Here's how the part is built. I have some questions about the finished solid (model axes, mm). A direction names the side the tool comes from. Give positions to 0.01 mm unless a question says otherwise; leave off trailing zeros. Write each loop counter-clockwise with the first axis right and the second up, starting at its lowest first coordinate (ties: lowest second). Pieces come first, ordered by that corner, then holes. Notation, with made-up numbers: (-4.5, -37.5) -> (49.5, -37.5) arc R9 ccw to (49.5, -26.5) -> close; hole circle Ø7 at (5, -8.75). An arc over 180 degrees is marked (long way). Return JSON: item names as keys, results as strings.
from build123d import *

# Parameters (mm, degrees)
F1_DEPTH  = 43.0059846
F4_DEPTH  = 44.9897246
F5_R      = 1.98374
F6_R      = 3.69316
F7_SIZE   = 33.4809846
F8_R      = 11.2530001
F8_R_2    = 1.5
F9_DEPTH  = 1.70942
F10_R     = 1.8288
F11_DEPTH = 1.70942
F12_R     = 0.762


with BuildPart() as f1:
    # F0 (on Top) → F1 (new body)
    with BuildSketch(Plane.XY):
        Polygon((-1.70942, 0), (0, 0), (0, 46.9734646), (46.9734646, 46.9734646), (46.9734646, 0), (48.6828846, 0), (48.6828846, 48.6828846), (-1.70942, 48.6828846), align=None)
    extrude(amount=F1_DEPTH)

    # F3 (on face) → F4 (join, through all)
    with BuildSketch(Plane.XZ):
        Polygon((48.6828846, 0), (46.9734646, 0), (46.9734646, -3.69316), (58.6041246, -3.69316), (58.6041246, -1.98374), (48.6828846, -1.98374), align=None)
        Polygon((0, 0), (-1.70942, 0), (-1.70942, -1.98374), (-11.63066, -1.98374), (-11.63066, -3.69316), (0, -3.69316), align=None)
    extrude(amount=-F4_DEPTH)

    # F5
    f5_edges = [f1.edges().sort_by_distance(p)[0] for p in [
        (0, 46.973465, 21.502992),
        (46.973465, 46.973465, 21.502992),
        (-1.70942, 22.494862, -1.98374),
        (48.682885, 22.494862, -1.98374),
    ]]
    fillet(f5_edges, radius=F5_R)

    # F6
    f6_edges = [f1.edges().sort_by_distance(p)[0] for p in [
        (48.682885, 48.682885, 21.502992),
        (-1.70942, 48.682885, 21.502992),
        (0, 22.494862, -3.69316),
        (46.973465, 22.494862, -3.69316),
    ]]
    fillet(f6_edges, radius=F6_R)

    # F7
    f7_edges = [f1.edges().sort_by_distance(p)[0] for p in [
        (-0.85471, 0, 43.005985),
        (47.828175, 0, 43.005985),
    ]]
    chamfer(f7_edges, length=F7_SIZE)

    # F8 (on face) → F9 (cut, through all)
    with BuildSketch(Plane.XZ.offset(-46.9734646)):
        with Locations((23.4867323, 21.5029923)):
            Circle(F8_R)
        with Locations((38.9867267, 37.0029867)):
            Circle(F8_R_2)
        with Locations((38.9867267, 6.0029979)):
            Circle(F8_R_2)
        with Locations((7.9867379, 6.0029979)):
            Circle(F8_R_2)
        with Locations((7.9867379, 37.0029867)):
            Circle(F8_R_2)
    extrude(amount=-F9_DEPTH, mode=Mode.SUBTRACT)

    # F10 (on face) → F11 (cut, through all)
    with BuildSketch(Plane(origin=(0, 0, -3.69316), x_dir=(1, 0, 0), z_dir=(0, 0, -1))):
        with Locations((54.6353746, -41.0209746001)):
            Circle(F10_R)
        with Locations((-7.66191, -41.0209746001)):
            Circle(F10_R)
        with Locations((-7.66191, -3.9687499999)):
            Circle(F10_R)
        with Locations((54.6353746, -3.9687499999)):
            Circle(F10_R)
    extrude(amount=-F11_DEPTH, mode=Mode.SUBTRACT)

    # F12
    f12_edges = [f1.edges().sort_by_distance(p)[0] for p in [
        (58.604125, 0, -2.83845),
        (-11.63066, 0, -2.83845),
        (-11.63066, 44.989725, -2.83845),
        (58.604125, 44.989725, -2.83845),
    ]]
    fillet(f12_edges, radius=F12_R)


solid = f1.part
1. Suppose I cut it at C-C, the plane x = 23. List the corners of the cut face in (y, z) for me.
Taken from the geometry:
{"outline": "(46.97, 0) -> (48.68, 0) -> (48.68, 10.26) -> (46.97, 10.26) -> close; (46.97, 32.75) -> (48.68, 32.75) -> (48.68, 43.01) -> (46.97, 43.01) -> close"}
2. If I drill on line 1 (X direction, y = 18, z = 9.5); line 2 (Y direction, x = 11, z = 19); line 3 (X direction, y = 25, z = -1.5) (3 decimals), over which ranges is the centre line in solid material (lowest first)? Write a range as [from, to].
Taken from the geometry:
{"line 1": "x = [-1.71, 0], [46.97, 48.68]", "line 2": "y = [46.97, 48.68]", "line 3": "x = [-2.395, -0.318], [47.292, 49.368]"}
3. If we mould it in two halves opening along X, with no side actions, what happens to faces 6 (the face through (-2.28, 22.81, -1.39)), 7 (the face through (37.49, 47.82, 6.07)), 8 (the face through (-8, 22, -1.984))? For each: released by +X, released by -X, zero draft, split by the parting line, or undercut.
Taken from the geometry:
{"face 6": "released by -X", "face 7": "undercut", "face 8": "zero draft"}
4. Suppose I cut it at D-D, the plane z = 1.5. List the corners of the cut face in (x, y) for me.
Taken from the geometry:
{"outline": "(-1.71, 0) -> (0, 0) -> (0, 44.99) arc R1.98 cw to (1.98, 46.97) -> (44.99, 46.97) arc R1.98 cw to (46.97, 44.99) -> (46.97, 0) -> (48.68, 0) -> (48.68, 44.99) arc R3.69 ccw to (44.99, 48.68) -> (1.98, 48.68) arc R3.69 ccw to (-1.71, 44.99) -> close"}
5. Suppose I cut it at A-A, the plane z = 14.5. List the corners of the cut face in (x, y) for me (3 decimals), and give its area (3 significant figures).
Taken from the geometry:
{"outline": "(-1.709, 4.975) -> (0, 4.975) -> (0, 44.99) arc R1.984 cw to (1.984, 46.973) -> (14.678, 46.973) -> (14.678, 48.683) -> (1.984, 48.683) arc R3.693 ccw to (-1.709, 44.99) -> close; (32.295, 46.973) -> (44.99, 46.973) arc R1.984 cw to (46.973, 44.99) -> (46.973, 4.975) -> (48.683, 4.975) -> (48.683, 44.99) arc R3.693 ccw to (44.99, 48.683) -> (32.295, 48.683) -> close", "area": "195 mm²"}
6. Suppose I cut it at B-B, the plane y = 17. List the corners of the cut face in (x, z) for me (3 decimals), and give its area (3 significant figures).
Taken from the geometry:
{"outline": "(-11.631, -3.693) -> (-3.693, -3.693) arc R3.693 ccw to (0, 0) -> (0, 26.525) -> (-1.709, 26.525) -> (-1.709, 0) arc R1.984 cw to (-3.693, -1.984) -> (-11.631, -1.984) -> close; (46.973, 0) arc R3.693 ccw to (50.667, -3.693) -> (58.604, -3.693) -> (58.604, -1.984) -> (50.667, -1.984) arc R1.984 cw to (48.683, 0) -> (48.683, 26.525) -> (46.973, 26.525) -> close", "area": "133 mm²"}
7. Which directions (+Z, -Z, +X, -X, +Y, -Y) give clear straight access to the entire face, cutting with the end or side of a thin tool? Please do faces 1 (the face through (-1.709, 28, 16)), 2 (the face through (46.973, 27, 17)), 3 (the face through (55, 22, -3.693)), 4 (the face through (-6, 44.99, -3)), 5 (the face through (-1.05, 22.81, -2.58)).
Taken from the geometry:
{"face 1": "+Z, -X, +Y, -Y", "face 2": "+Z, -Z, -Y", "face 3": "-Z, +X, -X, +Y, -Y", "face 4": "-Z, +X, -X, +Y", "face 5": "-Z, +Y, -Y"}
8. For pin 1 Ø12 at (y, z) = (18, 15) entering from +X; pin 2 Ø3 at (x, z) = (-6, -1) entering from +Y; pin 3 Ø10 at (x, z) = (22, 18.5) entering from -Y; pin 4 Ø10 at (x, z) = (51.5, 22.5) entering from +Y, each with a flat end and sliding along its axis, tell me the tip position at first contact or that it passes through.
Taken from the geometry:
{"pin 1": "stops at x = 48.68", "pin 2": "stops at y = 44.99", "pin 3": "passes through", "pin 4": "stops at y = 48.36"}
